Geometry: final body of the model. Coordinates: model frame, mm. A direction names the side the tool comes from. Round coordinates to 2 decimals unless told otherwise and drop trailing zeros. Loops run counter-clockwise (first coordinate to the right, second up) from the corner with the lowest first, then second, coordinate; pieces in that order, holes last. Notation, with made-up numbers: (60.5, 8.25) - (111.5, 8.25) arc R27 ccw to (111.5, 41.25) - close; hole circle Ø4 at (55.5, 8.5). An arc over 180 degrees is marked (long way). Use CSV: the item, a comma, the result in double quotes.
from build123d import *

# Parameters (mm, degrees)
F0_W        = 19.05
F0_H        = 19.05
F0_W_2      = 12.7
F0_H_2      = 12.7
F1_DEPTH    = 323.85
F3_T1_DEPTH = 66.675
F4_T1_DEPTH = 66.675
F2_R        = 3.175
F5_DEPTH    = 19.051
F2_R_2      = 4.7625
F6_DEPTH    = 3.175


# Not quite as in the source:
# - a fillet or chamfer that OpenCascade refuses, or shapes differently, is made with other operations: its cross-section is extruded or revolved along the edge and cut away or added


with BuildPart() as f1:
    # F0 (on Right) → F1 (new body)
    with BuildSketch(Plane.YZ):
        Rectangle(F0_W, F0_H)
        Rectangle(F0_W_2, F0_H_2, mode=Mode.SUBTRACT)
    extrude(amount=F1_DEPTH)

    # F3: fillet of radius 9.525 on 2 edges, made by hand

    # F3_s2 → F3_t1 (cut)
    with BuildSketch(Plane.XZ.offset(-33.3375)):
        with BuildLine():
            ThreePointArc((9.525, 9.525), (2.7898079092, 6.7351920908), (0, 0))
            Line((0, 0), (0, 9.525))
            Line((0, 9.525), (9.525, 9.525))
        make_face()
        with BuildLine():
            ThreePointArc((9.525, -9.525), (2.7898079092, -6.7351920908), (0, 0))
            Line((0, 0), (0, -9.525))
            Line((0, -9.525), (9.525, -9.525))
        make_face()
    extrude(amount=F3_T1_DEPTH, mode=Mode.SUBTRACT)

    # F4: fillet of radius 9.525 on 2 edges, made by hand

    # F4_s2 → F4_t1 (cut)
    with BuildSketch(Plane.XZ.offset(-33.3375)):
        with BuildLine():
            ThreePointArc((314.325, 9.525), (321.0601920908, 6.7351920908), (323.85, 0))
            Line((323.85, 0), (323.85, 9.525))
            Line((323.85, 9.525), (314.325, 9.525))
        make_face()
        with BuildLine():
            ThreePointArc((323.85, 0), (321.0601920908, -6.7351920908), (314.325, -9.525))
            Line((314.325, -9.525), (323.85, -9.525))
            Line((323.85, -9.525), (323.85, 0))
        make_face()
    extrude(amount=F4_T1_DEPTH, mode=Mode.SUBTRACT)

    # F2 (on face) → F5 (cut, through all)
    with BuildSketch(Plane.XZ.offset(9.525)):
        with Locations((314.325, 0)):
            Circle(F2_R)
        with Locations((161.925, 0)):
            Circle(F2_R)
        with Locations((9.525, 0)):
            Circle(F2_R)
    extrude(amount=-F5_DEPTH, mode=Mode.SUBTRACT)

    # F2 (on face) → F6 (cut, through all)
    with BuildSketch(Plane.XZ.offset(9.525)):
        with Locations((9.525, 0)):
            Circle(F2_R_2)
        with Locations((9.525, 0)):
            Circle(F2_R, mode=Mode.SUBTRACT)
        with Locations((161.925, 0)):
            Circle(F2_R_2)
        with Locations((161.925, 0)):
            Circle(F2_R, mode=Mode.SUBTRACT)
        with Locations((314.325, 0)):
            Circle(F2_R_2)
        with Locations((314.325, 0)):
            Circle(F2_R, mode=Mode.SUBTRACT)
    extrude(amount=-F6_DEPTH, mode=Mode.SUBTRACT)


solid = f1.part
Item 1: Pin query (flat end, axial travel): P1, Ø8.5, axis at x = 161.925, z = 0, coming from the -Y side; P2, Ø5, axis at y = 2, z = 5, coming from the +X side. Return the tip coordinate at first contact, or that it passes through.
Final values:
P1,"stops at y = 6.35"
P2,"stops at x = 321.42"
Item 2: Material intervals for line 1 (Y direction, x = 142.5, z = 4) (3 decimals); line 2 (X direction, y = 8, z = 8.5), sorted ascending.
Final values:
line 1,"y = -9.525 to -6.35, 6.35 to 9.525"
line 2,"x = 5.23 to 318.62"
Item 3: Section A-A on y = -3.75. Return the cut outline in (x, z) (3 decimals), plus the area to 3 significant figures.
Final values:
outline,"(2.425, -6.35) arc R9.525 ccw to (9.525, -9.525) - (314.325, -9.525) arc R9.525 ccw to (321.425, -6.35) - close; (2.425, 6.35) - (321.425, 6.35) arc R9.525 ccw to (314.325, 9.525) - (9.525, 9.525) arc R9.525 ccw to start"
area,"2,000 mm²"
Item 4: Section B-B on x = 53. Return the cut outline in (y, z) (3 decimals), plus the area to 3 significant figures.
Final values:
outline,"(-9.525, -9.525) - (9.525, -9.525) - (9.525, 9.525) - (-9.525, 9.525) - close; hole (-6.35, -6.35) - (6.35, -6.35) - (6.35, 6.35) - (-6.35, 6.35) - close"
area,"202 mm²"
Item 5: Reachability of faces 3 (the cylindrical face through (166.468, -7.96, 1.431)), 4 (the flat face through (160, 6.35, 3)), 5 (the flat face through (160, 0, -9.525)) from +Z, -Z, +X, -X, +Y, -Y: full face, straight path, thin tool, end or side. Return the list, or none.
Final values:
face 3,"-Y"
face 4,"+X, -X"
face 5,"-Z, +X, -X, +Y, -Y"
Item 6: Mould query, pull axis X, two halves, no side actions, for faces 1 (the cylindrical face through (12.458, 7.915, -1.216)), 2 (the flat face through (160, 0, -6.35)). Classes: released by +X, released by -X, zero draft, split by the parting line, or undercut.
Final values:
face 1,"undercut"
face 2,"zero draft"
